from build123d import *

# Parameters (mm, degrees)
SKETCH_1_W          = 10
SKETCH_1_H          = 10
SKETCH_1_W_2        = 8
SKETCH_1_H_2        = 8
EXTRUDE_1_DEPTH     = 65
SKETCH_2_R          = 1.5
CUT_EXTRUDE_1_DEPTH = 11
SKETCH_5_R          = 1.5
CUT_EXTRUDE_2_DEPTH = 11
CUT_EXTRUDE_START   = -5
SKETCH_6_R          = 3.5
CUT_EXTRUDE_3_DEPTH = 5


with BuildPart() as part:
    # 草图1 → 拉伸-薄壁1 (new body)
    with BuildSketch(Plane.XY):
        Rectangle(SKETCH_1_W, SKETCH_1_H)
        Rectangle(SKETCH_1_W_2, SKETCH_1_H_2, mode=Mode.SUBTRACT)
    extrude(amount=EXTRUDE_1_DEPTH)

    # 草图2 → 切除-拉伸1 (cut, through all)
    with BuildSketch(Plane.ZY.offset(5)):
        with Locations((40, 0)):
            Circle(SKETCH_2_R)
        with Locations((60, 0)):
            Circle(SKETCH_2_R)
        with Locations((5, 0)):
            Circle(SKETCH_2_R)
    extrude(amount=-CUT_EXTRUDE_1_DEPTH, mode=Mode.SUBTRACT)

    # 草图5 → 切除-拉伸2 (cut, through all)
    with BuildSketch(Plane(origin=(0, 5, 0), x_dir=(1, 0, 0), z_dir=(0, 1, 0))):
        with Locations((0, -10)):
            Circle(SKETCH_5_R)
        with Locations((0, -50)):
            Circle(SKETCH_5_R)
    extrude(amount=-CUT_EXTRUDE_2_DEPTH, mode=Mode.SUBTRACT)

    # 草图6 → 切除-拉伸3 (cut)
    with BuildSketch(Plane(origin=(0, 5, 0), x_dir=(1, 0, 0), z_dir=(0, 1, 0)).offset(CUT_EXTRUDE_START)):
        with Locations((0, -10)):
            Circle(SKETCH_6_R)
        with Locations((0, -50)):
            Circle(SKETCH_6_R)
    extrude(amount=-CUT_EXTRUDE_3_DEPTH, mode=Mode.SUBTRACT)


solid = part.part
Design review of the part built by this model. Coordinates are the model's own, in mm. A direction names the side the tool comes from. Give positions to 0.01 mm unless a question says otherwise; leave off trailing zeros. Order: outer loops, then holes, each group sorted by start corner. A loop starts at its lowest first (then second) coordinate and runs counter-clockwise, first axis right, second up.
1. Tool access review of faces 5 (the cylindrical face through (-0.325, 4.507, 51.464)), 6 (the cylindrical face through (-0.759, -4.493, 13.417)), 7 (the flat face through (-4, 0, 32)): name each direction out of +Z, -Z, +X, -X, +Y, -Y from which nothing blocks a thin tool from reaching the whole face with its end or side.
Solution:
face 5: +Y, -Y
face 6: -Y
face 7: +Z, -Z
2. Add section C-C, the plane y = 0. State how many separate pieces and enclosed holes the cut face has, then the cut area to 3 significant figures.
Solution:
separate pieces: 8
enclosed holes: 0
area: 112 mm2
3. Add section D-D, the plane x = 2.5. State the section outline as (y, z) points.
Solution:
outline: (-5, 0) - (-4, 0) - (-4, 7.55) - (-5, 7.55) - close; (-5, 12.45) - (-4, 12.45) - (-4, 47.55) - (-5, 47.55) - close; (-5, 52.45) - (-4, 52.45) - (-4, 65) - (-5, 65) - close; (4, 0) - (5, 0) - (5, 65) - (4, 65) - close
4. Add section B-B, the plane z = 50. State the section outline as (x, y) points.
Solution:
outline: (-5, -5) - (-3.5, -5) - (-3.5, -4) - (-4, -4) - (-4, 4) - (-1.5, 4) - (-1.5, 5) - (-5, 5) - close; (1.5, 4) - (4, 4) - (4, -4) - (3.5, -4) - (3.5, -5) - (5, -5) - (5, 5) - (1.5, 5) - close
5. To check wall thickness, follow L1, parallel to Z at x = 0, y = -4.3; L2, parallel to Z at x = 0, y = 4.75; L3, parallel to X at y = -2.25, z = 18. State the ranges of each line that lie inside material, in increasing order.
Solution:
L1: z = 0 to 6.5, 13.5 to 46.5, 53.5 to 65
L2: z = 0 to 8.5, 11.5 to 48.5, 51.5 to 65
L3: x = -5 to -4, 4 to 5
6. Add section A-A, the plane x = 0. State the section outline as (y, z) points, then the cut area to 3 significant figures.
Solution:
outline: (-5, 0) - (-4, 0) - (-4, 6.5) - (-5, 6.5) - close; (-5, 13.5) - (-4, 13.5) - (-4, 46.5) - (-5, 46.5) - close; (-5, 53.5) - (-4, 53.5) - (-4, 65) - (-5, 65) - close; (4, 0) - (5, 0) - (5, 8.5) - (4, 8.5) - close; (4, 11.5) - (5, 11.5) - (5, 48.5) - (4, 48.5) - close; (4, 51.5) - (5, 51.5) - (5, 65) - (4, 65) - close
area: 110 mm2
7. Mouldability with a two-part tool opening along Y and no side actions: class faces 1 (the flat face through (0, 5, 32)), 2 (the flat face through (5, 0, 32)), 3 (the cylindrical face through (4.493, -0.575, 6.386)), 4 (the flat face through (0, 4, 32)) as +Y half, -Y half, draft (parallel to the pull), parting line (faces both ways), or undercut.
Solution:
face 1: +Y half
face 2: draft
face 3: undercut
face 4: undercut
